Here's how the part is built. I have some questions about the finished solid (model axes, mm). Face numbers are marked on the shaded views. A direction names the side the tool comes from. Round coordinates to 2 decimals unless told otherwise and drop trailing zeros. Write each loop counter-clockwise with the first axis right and the second up, starting at its lowest first coordinate (ties: lowest second). Pieces come first, ordered by that corner, then holes. Notation, with made-up numbers: M 84,9.5 L 133,9.5 A22 cw 133,42.5 Z; hole C 53.25,-13 d5. An arc over 180 degrees is marked long. Write item = value, one per line. Start each with the question number.
(1) I need wall thicknesses on line 1 along X through (y, z) = (-3, 12.5); line 2 along X through (y, z) = (-5.25, 75); line 3 along Y through (x, z) = (-74, 30). Which ranges of each line are inside material? Lowest first, please.
(2) I want a section at C-C (z = -24). List the corners of the cut face in (x, y) for me, and give its area (3 significant figures).
(3) I want a section at B-B (y = -5.5). Give the number of separate pieces and of enclosed holes in the cut face, and give its area (3 significant figures).
(4) On a 3-axis mill with a long thin cutter (end or side, diameter ignored), from which of +Z, -Z, +X, -X, +Y, -Y can I reach the whole of each face in a straight line? I mean the marked faces 1 and 2. Say none if no direction works.
(5) Will these pins go through, and if not, where does the flat tip stop? pin 1 Ø5 at (x, z) = (-82.5, -12.5) entering from +Y; pin 2 Ø6 at (x, y) = (55.5, -5) entering from +Z.
(6) I want a section at A-A (x = -46.5). List the corners of the cut face in (y, z) for me, and give its area (3 significant figures).
```python
from build123d import *

# Parameters (mm, degrees)
MAIN_DEPTH                      = 107.5
F_4_0MM_DOWEL_HOLE1_D           = 4.1
F_4_0MM_DOWEL_HOLE1_ON_FACE_2_D = 4.1
F_4_0MM_DOWEL_HOLE1_ON_FACE_3_D = 4.1
F_4_0MM_DOWEL_HOLE1_ON_FACE_4_D = 4.1
SKETCH4_R                       = 1.6
ATTACHMENT_SCREW_HOLES_DEPTH    = 151.392275662


with BuildPart() as part:
    # Sketch2 → Main (new, symmetric)
    with BuildSketch(Plane(origin=(0, 0, 0), x_dir=(0, 0, -1), z_dir=(1, 0, 0))):
        Polygon((-85, 0), (85, 0), (97.5, 12.5), (103.156854249, 6.843145751), (88.313708499, -8), (-88.313708499, -8), (-103.156854249, 6.843145751), (-97.5, 12.5), align=None)
    extrude(amount=MAIN_DEPTH, both=True)

    # Ø4.0mm Dowel Hole1 (through all)
    with Locations(Plane(origin=(-102.5, 7.071067812, -92.071067812), x_dir=(0, 0.707106781187, -0.707106781187), z_dir=(0, 0.707106781187, 0.707106781187))):
        with Locations((0, 0)):
            Hole(F_4_0MM_DOWEL_HOLE1_D / 2)

    # Ø4.0mm Dowel Hole1 on face 2 (through all)
    with Locations(Plane(origin=(-102.5, 0, -75), x_dir=(0, 0, 1), z_dir=(0, 1, 0))):
        with Locations((0, 0), (75, 0), (150, 0), (150, 205), (75, 205), (0, 205)):
            Hole(F_4_0MM_DOWEL_HOLE1_ON_FACE_2_D / 2)

    # Ø4.0mm Dowel Hole1 on face 3 (through all)
    with Locations(Plane(origin=(-102.5, 7.071067812, 92.071067812), x_dir=(0, -0.707106781187, -0.707106781187), z_dir=(0, 0.707106781187, -0.707106781187))):
        with Locations((0, 0), (0, -205)):
            Hole(F_4_0MM_DOWEL_HOLE1_ON_FACE_3_D / 2)

    # Ø4.0mm Dowel Hole1 on face 4 (through all)
    with Locations(Plane(origin=(102.5, 7.071067812, -92.071067812), x_dir=(0, 0.707106781187, -0.707106781187), z_dir=(0, 0.707106781187, 0.707106781187))):
        with Locations((0, 0)):
            Hole(F_4_0MM_DOWEL_HOLE1_ON_FACE_4_D / 2)

    # Sketch4 → Attachment screw holes (cut, through all)
    with BuildSketch(Plane.XZ.offset(8)):
        with Locations(Location((57.5, 12.5, 0), (0, 0, 270))):
            Circle(SKETCH4_R)
        with Locations(Location((82.5, 12.5, 0), (0, 0, 270))):
            Circle(SKETCH4_R)
        with Locations(Location((82.5, -12.5, 0), (0, 0, 270))):
            Circle(SKETCH4_R)
        with Locations(Location((57.5, -12.5, 0), (0, 0, 270))):
            Circle(SKETCH4_R)
    attachment_screw_holes = extrude(amount=-ATTACHMENT_SCREW_HOLES_DEPTH, mode=Mode.SUBTRACT)

    # Mirror1: Attachment screw holes across plane
    add(attachment_screw_holes.mirror(Plane(origin=(0, 0, 0), x_dir=(0, 0, 1), z_dir=(1, 0, 0))), mode=Mode.SUBTRACT)


solid = part.part
```
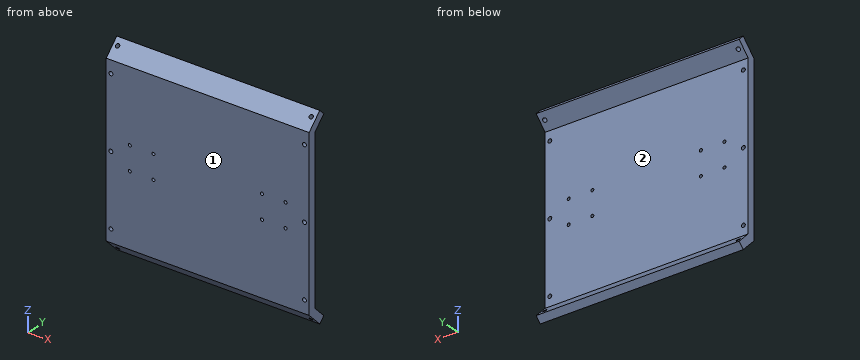
Returned:
q1.line_1 = -107.5 to -84.1, -80.9 to -59.1, -55.9 to 55.9, 59.1 to 80.9, 84.1 to 107.5
q1.line_2 = -107.5 to -104.55, -100.45 to 100.45, 104.55 to 107.5
q1.line_3 = -8 to 0
q2.outline = M -107.5,-8 L 107.5,-8 L 107.5,0 L -107.5,0 Z
q2.area = 1,720 mm²
q3.separate_pieces = 1
q3.enclosed_holes = 14
q3.area = 38,900 mm²
q4.face_1 = +Z, -Z, +X, -X, -Y
q4.face_2 = +X, -X, +Y
q5.pin_1 = 0
q5.pin_2 = 94.31
q6.outline = M -8,-88.31 L 6.84,-103.16 L 12.5,-97.5 L 0,-85 L 0,85 L 12.5,97.5 L 6.84,103.16 L -8,88.31 Z
q6.area = 1,700 mm²
